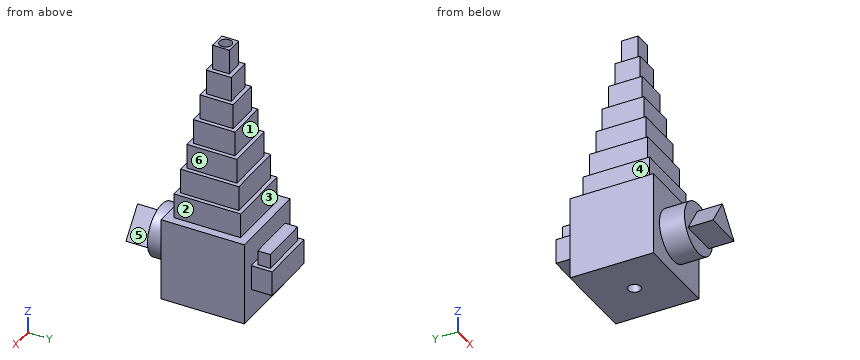
from build123d import *

# Parameters (mm, degrees)
F0_W      = 254
F0_H      = 254
F1_DEPTH  = 254
F3_W      = 203.2
F3_H      = 203.2
F4_DEPTH  = 76.2
F5_W      = 177.8
F5_H      = 177.8
F6_DEPTH  = 76.2
F7_W      = 152.4
F7_H      = 152.4
F8_DEPTH  = 76.2
F9_W      = 127
F9_H      = 127
F10_DEPTH = 76.2
F11_W     = 101.6
F11_H     = 101.6
F12_DEPTH = 76.2
F13_W     = 76.2
F13_H     = 76.2
F14_DEPTH = 76.2
F15_W     = 50.8
F15_H     = 50.8
F16_DEPTH = 76.2
F18_D     = 38.1
F2_R      = 78.384175
F19_DEPTH = 76.2
F21_DEPTH = 76.2
F22_W     = 177.8
F22_H     = 76.2
F23_DEPTH = 63.5
F25_W     = 152.4
F25_H     = 38.1
F26_DEPTH = 44.45


with BuildPart() as f1:
    # F0 (on Front) → F1 (new body)
    with BuildSketch(Plane.XZ):
        with Locations((32.72583, 38.734609)):
            Rectangle(F0_W, F0_H)
    extrude(amount=F1_DEPTH)

    # F3 (on face) → F4 (join)
    with BuildSketch(Plane.XY.offset(165.734609)):
        with Locations((32.72583, -127)):
            Rectangle(F3_W, F3_H)
    extrude(amount=F4_DEPTH)

    # F5 (on face) → F6 (join)
    with BuildSketch(Plane.XY.offset(241.934609)):
        with Locations((32.72583, -127)):
            Rectangle(F5_W, F5_H)
    extrude(amount=F6_DEPTH)

    # F7 (on face) → F8 (join)
    with BuildSketch(Plane.XY.offset(318.134609)):
        with Locations((32.72583, -127)):
            Rectangle(F7_W, F7_H)
    extrude(amount=F8_DEPTH)

    # F9 (on face) → F10 (join)
    with BuildSketch(Plane.XY.offset(394.334609)):
        with Locations((32.72583, -127)):
            Rectangle(F9_W, F9_H)
    extrude(amount=F10_DEPTH)

    # F11 (on face) → F12 (join)
    with BuildSketch(Plane.XY.offset(470.534609)):
        with Locations((32.72583, -127)):
            Rectangle(F11_W, F11_H)
    extrude(amount=F12_DEPTH)

    # F13 (on face) → F14 (join)
    with BuildSketch(Plane.XY.offset(546.734609)):
        with Locations((32.72583, -127)):
            Rectangle(F13_W, F13_H)
    extrude(amount=F14_DEPTH)

    # F15 (on face) → F16 (join)
    with BuildSketch(Plane.XY.offset(622.934609)):
        with Locations((32.725834, -127)):
            Rectangle(F15_W, F15_H)
    extrude(amount=F16_DEPTH)

    # F18 (through all)
    with Locations(Plane.XY.offset(699.134609)):
        with Locations((32.725834, -127)):
            Hole(F18_D / 2)

    # F2 (on face) → F19 (join)
    with BuildSketch(Plane.XZ.offset(254)):
        with Locations((18.441331, 29.720267)):
            Circle(F2_R)
    extrude(amount=F19_DEPTH)

    # F20 (on face) → F21 (join)
    with BuildSketch(Plane.XZ.offset(330.2)):
        Polygon((77.017064, 0), (12.2257, 82.338598), (-40.134403, 0), align=None)
    extrude(amount=F21_DEPTH)

    # F22 (on face) → F23 (join)
    with BuildSketch(Plane(origin=(0, 0, 0), x_dir=(-1, 0, 0), z_dir=(0, 1, 0))):
        with Locations((-32.72583, 38.734609)):
            Rectangle(F22_W, F22_H)
    extrude(amount=F23_DEPTH)

    # F25 (on face) → F26 (join)
    with BuildSketch(Plane.XY.offset(76.834609)):
        with Locations((32.72583, 31.75)):
            Rectangle(F25_W, F25_H)
    extrude(amount=F26_DEPTH)


solid = f1.part
Input: part model. Units: mm. Frame: model coordinates. Face numbers are marked on the shaded views. A direction names the side the tool comes from. Coordinates: 2 decimals unless noted, no trailing zeros. Order: outer loops, then holes, each group sorted by start corner. A loop starts at its lowest first (then second) coordinate and runs counter-clockwise, first axis right, second up.
1. Access query for the marked faces 3, 4, 5 and 6. Directions: +Z, -Z, +X, -X, +Y, -Y. A direction counts if a zero-diameter tool reaches every point of the face in a straight line with its end or side. Return the directions, or none.
Checked values:
face 3: +Z, +X, -X, +Y
face 4: +Z, -X, +Y, -Y
face 5: +Z, +X, -Y
face 6: +Z, +X, +Y, -Y
2. Ray query, line 1 along Y through (x, z) = (31, 635.5); line 2 along Z through (x, y) = (-47, -222.5); line 3 along Z through (x, y) = (16, -244). Return the intervals inside material, ascending.
Checked values:
line 1: y = -152.4 to -145.97, -108.03 to -101.6
line 2: z = -88.27 to 241.93
line 3: z = -88.27 to 165.73
3. Draft query along Y for the marked faces 1 and 2. Return one class per face: +Y half, -Y half, draft (parallel to the pull), parting line (faces both ways), or undercut.
Checked values:
face 1: +Y half
face 2: draft
4. Cut plane A-A, the plane z = 157.5. Return loops of the section in (x, y), plus the area to 3 significant figures.
Checked values:
outline: (-94.27, -254) - (159.73, -254) - (159.73, 0) - (-94.27, 0) - close; hole circle Ø38.1 at (32.73, -127)
area: 63,400 mm2
5. Contact query for flat-ended pins moving along their axis: P1, Ø2, axis at x = 121, y = -213, coming from the +Z side; P2, Ø23, axis at y = -107, z = 202.5, coming from the +X side; P3, Ø23, axis at x = 67, z = 214, coming from the +Y side. Output: stop coordinate, or through.
Checked values:
P1: stops at z = 318.13
P2: stops at x = 134.33
P3: stops at y = -25.4
6. Cut plane D-D, the plane y = -238. Return loops of the section in (x, z), plus the area to 3 significant figures.
Checked values:
outline: (-94.27, -88.27) - (159.73, -88.27) - (159.73, 165.73) - (-94.27, 165.73) - close
area: 64,500 mm2
7. Cut plane C-C, the plane z = 21.5. Return loops of the section in (x, y), plus the area to 3 significant figures.
Checked values:
outline: (-94.27, -254) - (-59.51, -254) - (-59.51, -330.2) - (-26.46, -330.2) - (-26.46, -406.4) - (60.1, -406.4) - (60.1, -330.2) - (96.39, -330.2) - (96.39, -254) - (159.73, -254) - (159.73, 0) - (121.63, 0) - (121.63, 63.5) - (-56.17, 63.5) - (-56.17, 0) - (-94.27, 0) - close; hole circle Ø38.1 at (32.73, -127)
area: 93,100 mm2
8. Cut plane B-B, the plane y = 30. Return loops of the section in (x, z), plus the area to 3 significant figures.
Checked values:
outline: (-56.17, 0.63) - (121.63, 0.63) - (121.63, 76.83) - (108.93, 76.83) - (108.93, 121.28) - (-43.47, 121.28) - (-43.47, 76.83) - (-56.17, 76.83) - close
area: 20,300 mm2
